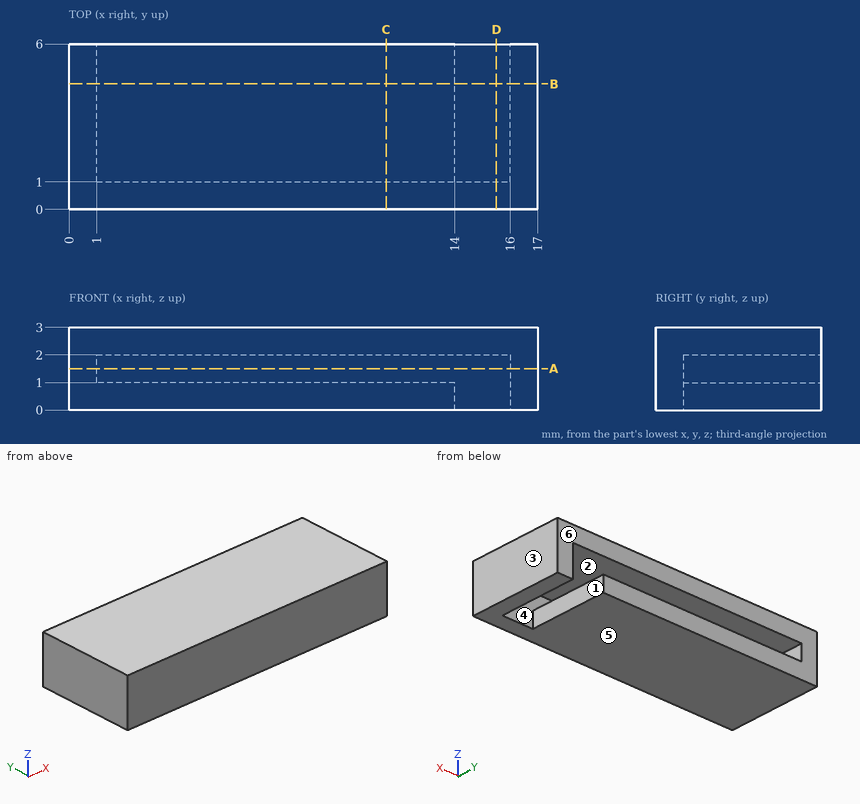
Source: three-view drawing plus pictorial views. Frame: mm from the lowest corner of the part. A direction names the side the tool comes from. Round coordinates to 2 decimals unless told otherwise and drop trailing zeros. Write each loop counter-clockwise with the first axis right and the second up, starting at its lowest first coordinate (ties: lowest second). Pieces come first, ordered by that corner, then holes. Notation, with made-up numbers: (-31.75, 16.5) -> (-25.75, 16.5) arc R8 ccw to (-25.75, 29.5) -> close; hole circle Ø10 at (80, 47). An arc over 180 degrees is marked (long way). Return JSON: item names as keys, results as strings.
Q1. Section B-B on y = 4.55. Return the cut outline in (x, z), and give its area (3 significant figures).
From the geometry:
{"outline": "(0, 0) -> (14, 0) -> (14, 1) -> (1, 1) -> (1, 2) -> (16, 2) -> (16, 0) -> (17, 0) -> (17, 3) -> (0, 3) -> close", "area": "34.0 mm2"}
Q2. Ray query, line 1 (X direction, y = 4.25, z = 0.9); line 2 (Z direction, x = 5, y = 3.1); line 3 (X direction, y = 1.95, z = 1.5). Return the intervals inside material, ascending.
From the geometry:
{"line 1": "0 to 14, 16 to 17", "line 2": "0 to 1, 2 to 3", "line 3": "0 to 1, 16 to 17"}
Q3. Mould query, pull axis Z, two halves, no side actions, for the marked faces 4, 5 and 6. Classes: +Z half, -Z half, draft (parallel to the pull), parting line (faces both ways), or undercut.
From the geometry:
{"face 4": "undercut", "face 5": "-Z half", "face 6": "draft"}
Q4. Section A-A on z = 1.5. Return the cut outline in (x, y), and give its area (3 significant figures).
From the geometry:
{"outline": "(0, 0) -> (17, 0) -> (17, 6) -> (16, 6) -> (16, 1) -> (1, 1) -> (1, 6) -> (0, 6) -> close", "area": "27.0 mm2"}
Q5. Section D-D on x = 15.5. Return the cut outline in (y, z), and give its area (3 significant figures).
From the geometry:
{"outline": "(0, 0) -> (1, 0) -> (1, 2) -> (6, 2) -> (6, 3) -> (0, 3) -> close", "area": "8.00 mm2"}
Q6. Set-up query: the marked faces 1, 2 and 3. Return all of +Z, -Z, +X, -X, +Y, -Y with unobstructed straight access to the full face (end or side cutting, diameter ignored); none if empty.
From the geometry:
{"face 1": "-Z, +Y", "face 2": "+Y", "face 3": "+Z, -Z, +X, +Y, -Y"}
Q7. Section C-C on x = 11.5. Return the cut outline in (y, z).
From the geometry:
{"outline": "(0, 0) -> (6, 0) -> (6, 1) -> (1, 1) -> (1, 2) -> (6, 2) -> (6, 3) -> (0, 3) -> close"}
